```python
from build123d import *

# Parameters (mm, degrees)
F1_DEPTH = 12.7
F2_R     = 2.54
F3_R     = 0.127
F4_R     = 3.3782
F5_DEPTH = 6.351
F6_R     = 3.3782
F7_DEPTH = 6.351


with BuildPart() as f1:
    # F0 (on Front) → F1 (new body, symmetric)
    with BuildSketch(Plane.XZ):
        Polygon((6.35, 44.45), (0, 44.45), (0, 3.175), (0, 0), (0, -3.175), (31.75, -3.175), (31.75, 3.175), (6.35, 3.175), align=None)
    extrude(amount=F1_DEPTH, both=True)

    # F2
    f2_edges = [f1.edges().sort_by_distance(p)[0] for p in [
        (6.35, 0, 3.175),
    ]]
    fillet(f2_edges, radius=F2_R)

    # F3
    f3_edges = [f1.edges().sort_by_distance(p)[0] for p in [
        (6.35, 0, 44.45),
        (0, 0, 44.45),
        (3.175, -12.7, 44.45),
        (6.35, -12.7, 25.0825),
        (20.32, -12.7, 3.175),
        (15.875, -12.7, -3.175),
        (0, -12.7, 20.6375),
        (31.75, 0, 3.175),
        (31.75, 0, -3.175),
        (20.32, 12.7, 3.175),
        (31.75, 12.7, 0),
        (15.875, 12.7, -3.175),
        (0, 12.7, 20.6375),
        (6.35, 12.7, 25.0825),
        (0, 0, -3.175),
        (31.75, -12.7, 0),
        (3.175, 12.7, 44.45),
    ]]
    fillet(f3_edges, radius=F3_R)

    # F4 (on face) → F5 (cut, through all)
    with BuildSketch(Plane.YZ.offset(6.35)):
        with Locations((-6.35, 31.75)):
            Circle(F4_R)
        with Locations((6.35, 31.75)):
            Circle(F4_R)
    extrude(amount=-F5_DEPTH, mode=Mode.SUBTRACT)

    # F6 (on face) → F7 (cut, through all)
    with BuildSketch(Plane.XY.offset(3.175)):
        with Locations((22.733, 0)):
            Circle(F6_R)
    extrude(amount=-F7_DEPTH, mode=Mode.SUBTRACT)


solid = f1.part
```
CAD build for the part. Positions are in the model's coordinates, mm. A direction names the side the tool comes from. Round coordinates to 2 decimals unless told otherwise and drop trailing zeros. Write each loop counter-clockwise with the first axis right and the second up, starting at its lowest first coordinate (ties: lowest second). Pieces come first, ordered by that corner, then holes. Notation, with made-up numbers: (-19, -38.5) - (23, -38.5) arc R20 cw to (23, -15.5) - close; hole circle Ø9 at (-11, -3.5). An arc over 180 degrees is marked (long way). Return JSON: item names as keys, results as strings. Group by question number.
Item 1: Band-saw the part on C-C on z = 6.5. List the corners of the cut face in (x, y).
Item 2: 3-axis set-ups, long thin cutter, end or side, ignore diameter. For faces 1 (the face through (3, 0, 44.45)), 2 (the face through (18, 0, 3.175)): which of +Z, -Z, +X, -X, +Y, -Y reach the whole face in a straight line?
Item 3: Flat gauge pins, fed straight in: pin 1 Ø12 at (x, z) = (14, 13.5) entering from +Y; pin 2 Ø7.5 at (y, z) = (2, 29) entering from +X; pin 3 Ø3 at (x, y) = (25.5, -2.5) entering from +Z (3 decimals). Where does each tip first touch, or does it go through?
Item 4: Mould opens along Y. For faces 3 (the face through (3.219, 7.909, 28.753)), 4 (the face through (5, 12.7, 15)), 5 (the face through (7.074, 0.176, 3.939)) say: +Y half, -Y half, draft (parallel to the pull), parting line (faces both ways), or undercut.
Item 5: Band-saw the part on A-A on y = 0. List the corners of the cut face in (x, z) (3 decimals).
Item 6: Probe probe 1 along Z at (x, y) = (3.75, -6.35) (3 decimals); probe 2 along Y at (x, z) = (3, 31.5); probe 3 along X at (y, z) = (-2, 32). List the from-to ranges inside material, lowest first.
Item 7: Band-saw the part on D-D on z = 31.75. List the corners of the cut face in (x, y).
Item 8: Band-saw the part on B-B on x = 17. List the corners of the cut face in (y, z) (3 decimals), plus the area to 3 significant figures.
Resolved:
{
 "1": {"outline": "(0, -12.57) arc R0.13 ccw to (0.13, -12.7) - (6.22, -12.7) arc R0.13 ccw to (6.35, -12.57) - (6.35, 12.57) arc R0.13 ccw to (6.22, 12.7) - (0.13, 12.7) arc R0.13 ccw to (0, 12.57) - close"},
 "2": {"face 1": "+Z, +X, -X, +Y, -Y", "face 2": "+Z, +X, +Y, -Y"},
 "3": {"pin 1": "passes through", "pin 2": "stops at x = 6.35", "pin 3": "stops at z = 3.175"},
 "4": {"face 3": "undercut", "face 4": "+Y half", "face 5": "draft"},
 "5": {"outline": "(0, -3.048) arc R0.127 ccw to (0.127, -3.175) - (19.355, -3.175) - (19.355, 3.175) - (8.89, 3.175) arc R2.54 cw to (6.35, 5.715) - (6.35, 44.323) arc R0.127 ccw to (6.223, 44.45) - (0.127, 44.45) arc R0.127 ccw to (0, 44.323) - close; (26.111, -3.175) - (31.623, -3.175) arc R0.127 ccw to (31.75, -3.048) - (31.75, 3.048) arc R0.127 ccw to (31.623, 3.175) - (26.111, 3.175) - close"},
 "6": {"probe 1": "z = -3.175 to 28.372, 35.128 to 44.45", "probe 2": "y = -12.7 to -9.72, -2.98 to 2.98, 9.72 to 12.7", "probe 3": "x = 0 to 6.35"},
 "7": {"outline": "(0, -12.57) arc R0.13 ccw to (0.13, -12.7) - (6.22, -12.7) arc R0.13 ccw to (6.35, -12.57) - (6.35, -9.73) - (0, -9.73) - close; (0, -2.97) - (6.35, -2.97) - (6.35, 2.97) - (0, 2.97) - close; (0, 9.73) - (6.35, 9.73) - (6.35, 12.57) arc R0.13 ccw to (6.22, 12.7) - (0.13, 12.7) arc R0.13 ccw to (0, 12.57) - close"},
 "8": {"outline": "(-12.7, -3.048) arc R0.127 ccw to (-12.573, -3.175) - (12.573, -3.175) arc R0.127 ccw to (12.7, -3.048) - (12.7, 3.048) arc R0.127 ccw to (12.573, 3.175) - (-12.573, 3.175) arc R0.127 ccw to (-12.7, 3.048) - close", "area": "161 mm²"}
}
